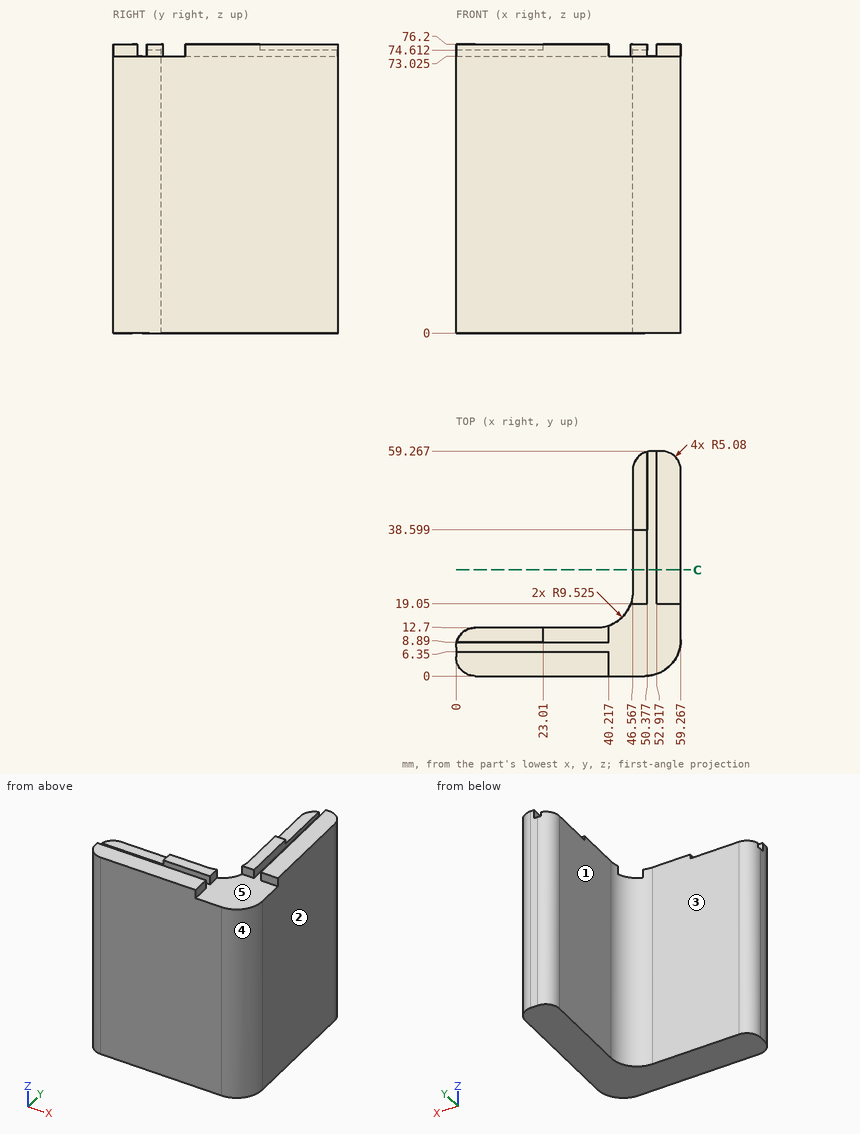
Check sheet for the drawn part. Datum: minimum x, y, z corner. Units: mm. A direction names the side the tool comes from. Coordinates: 2 decimals unless noted, no trailing zeros. Write each loop counter-clockwise with the first axis right and the second up, starting at its lowest first coordinate (ties: lowest second). Pieces come first, ordered by that corner, then holes. Notation, with made-up numbers: M -10.75,30 L 2.25,30 A9 cw 2.25,37 Z; hole C 29.25,70.5 d3. An arc over 180 degrees is marked long. One line per item, written item: value.
Item 1: Access from +Z, -Z, +X, -X, +Y, -Y to the whole of each face (thin tool, end or side, straight path). Record for the marked faces 1 and 2.
Check sheet entries:
face 1: +Z, -Z, -X, +Y
face 2: +Z, -Z, +X, +Y, -Y
Item 2: Scan lines: line 1 along Y through (x, z) = (30.5, 22.5); line 2 along X through (y, z) = (28, 33); line 3 along Z through (x, y) = (51.5, 21.5) (1 decimal). Record each from-to range of solid material in increasing order.
Check sheet entries:
line 1: y = 0 to 12.7
line 2: x = 46.57 to 59.27
line 3: z = 0 to 73
Item 3: Mould release check, pull along X, two halves, no side actions. Record for the marked faces 3, 4 and 5: pulls with the +X half, pulls with the -X half, needs draft (parallel to the pull), parting line crosses it, or undercut.
Check sheet entries:
face 3: needs draft
face 4: pulls with the +X half
face 5: undercut
Item 4: Gauge pin test, flat ends, axial feed: pin 1 Ø1.3 at (y, z) = (11, 75) entering from -X; pin 2 Ø2.5 at (x, z) = (28.5, 74.5) entering from +Y; pin 3 Ø2.5 at (y, z) = (11.5, 74) entering from +X; pin 4 Ø10 at (y, z) = (41.5, 43) entering from -X. Record the tip position at first contact, or that the pin passes through.
Check sheet entries:
pin 1: stops at x = 0.88
pin 2: stops at y = 12.7
pin 3: stops at x = 59.27
pin 4: stops at x = 46.57
Item 5: Section check C-C, the plane y = 28. Record the boundary of the cut face in (x, z) (1 decimal).
Check sheet entries:
outline: M 46.6,0 L 59.3,0 L 59.3,76.2 L 52.9,76.2 L 52.9,73 L 50.4,73 L 50.4,76.2 L 46.6,76.2 Z
